Work out the finished part from the listing and answer in its coordinate system (mm). Face numbers are marked on the shaded views. A direction names the side the tool comes from. Coordinates: 2 decimals unless noted, no trailing zeros. Order: outer loops, then holes, each group sorted by start corner. A loop starts at its lowest first (then second) coordinate and runs counter-clockwise, first axis right, second up. Notation, with made-up numbers: (67, 25.25) -> (77, 25.25) arc R15 cw to (77, 37.25) -> close; hole circle Ø4 at (44, 7). An arc over 180 degrees is marked (long way). Answer as CSV lines item,"result". Start each with the question number.
Item 1: Straight lines are drawn through the part: L1, parallel to X at y = 2, z = 28; L2, parallel to Y at x = -7, z = 18.75; L3, parallel to X at y = 5, z = 4. For each, find the intervals that lie inside material, in ascending order.
Item 2: Section A-A (y = 0) is taken. Write down the section's boundary in (x, z).
Item 3: Each of these flat-tipped pins is pushed along its axis until it touches: pin 1 Ø16.5 at (y, z) = (-4, 21) entering from +X; pin 2 Ø1.5 at (y, z) = (-15.5, 19) entering from -X; pin 3 Ø4.5 at (y, z) = (-7, 8.5) entering from -X. Where does it stop, or does it pass through?
Item 4: Section C-C (z = 7.25) is taken. Count the separate pieces of the cut face and the enclosed holes in it, then the cut area to 3 significant figures.
Item 5: Which of the six approach directions +Z, -Z, +X, -X, +Y, -Y give full straight-line access (tool end or side, diameter ignored) to the marked faces 4, 5 and 6?
Item 6: For a pull along X with two mould halves and no side action, classify the marked faces 1, 2 and 3 as pulls with the +X half, pulls with the -X half, needs draft (parallel to the pull), parting line crosses it, or undercut.
Item 7: Section D-D (y = -15) is taken. Write down the section's boundary in (x, z), then the cut area to 3 significant figures.
Item 8: Section B-B (x = -5) is taken. Write down the section's boundary in (y, z), then the cut area to 3 significant figures.
```python
from build123d import *

# Parameters (mm, degrees)
SKETCH_1_W      = 15
SKETCH_1_H      = 25.166666667
EXTRUDE_1_DEPTH = 30
FILLET_1_R      = 5
FILLET_2_R      = 5
FILLET_3_R      = 5


with BuildPart() as part:
    # 草圖1 → 填料-伸長1 (new body)
    with BuildSketch(Plane.XY):
        Polygon((-23.5, 11.416666667), (51.5, 11.416666667), (51.5, 8.416666667), (46.5, 8.416666667), (46.5, -16.75), (51.5, -16.75), (51.5, -19.75), (-23.5, -19.75), (-23.5, -17.25), (-18.5, -17.25), (-18.5, 7.916666667), (-23.5, 7.916666667), align=None)
        with Locations((-6, -4.166666666)):
            Rectangle(SKETCH_1_W, SKETCH_1_H, mode=Mode.SUBTRACT)
        with Locations((14, -4.166666666)):
            Rectangle(SKETCH_1_W, SKETCH_1_H, mode=Mode.SUBTRACT)
        with Locations((34, -4.166666666)):
            Rectangle(SKETCH_1_W, SKETCH_1_H, mode=Mode.SUBTRACT)
    extrude(amount=EXTRUDE_1_DEPTH)

    # 圓角1
    fillet_1_edges = [part.edges().sort_by_distance(p)[0] for p in [
        (-18.5, 7.916666667, 15),
    ]]
    fillet(fillet_1_edges, radius=FILLET_1_R - 0.0001)  # a hair under: the kernel refuses the full size

    # 圓角2
    fillet_2_edges = [part.edges().sort_by_distance(p)[0] for p in [
        (-18.5, -17.25, 15),
    ]]
    fillet(fillet_2_edges, radius=FILLET_2_R - 0.0001)  # a hair under: the kernel refuses the full size

    # 圓角3
    fillet_3_edges = [part.edges().sort_by_distance(p)[0] for p in [
        (46.5, 8.416666667, 15),
        (46.5, -16.75, 15),
        (-13.5, 8.416666667, 15),
        (-13.5, -16.75, 15),
        (1.5, -16.75, 15),
        (1.5, 8.416666667, 15),
        (6.5, 8.416666667, 15),
        (6.5, -16.75, 15),
        (21.5, -16.75, 15),
        (21.5, 8.416666667, 15),
        (26.5, 8.416666667, 15),
        (26.5, -16.75, 15),
        (41.5, -16.75, 15),
        (41.5, 8.416666667, 15),
    ]]
    fillet(fillet_3_edges, radius=FILLET_3_R - 0.0001)  # a hair under: the kernel refuses the full size


solid = part.part
```
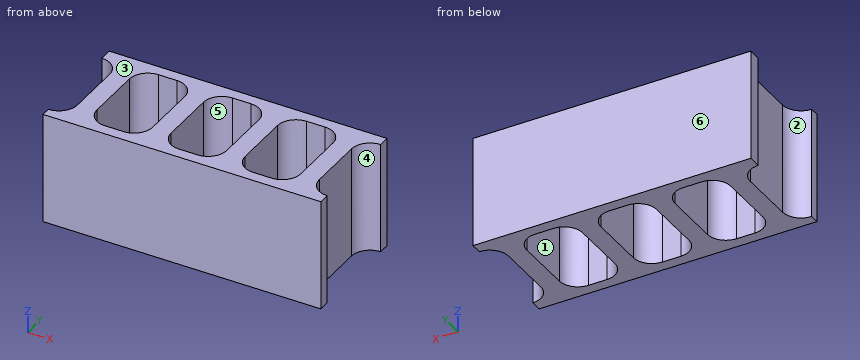
Checked values:
1,L1,"x = -18.5 to -13.5, 1.5 to 6.5, 21.5 to 26.5, 41.5 to 46.5"
1,L2,"y = -19.75 to -16.75, 8.42 to 11.42"
1,L3,"x = -18.95 to -13.24, 1.24 to 6.76, 21.24 to 26.76, 41.24 to 46.76"
2,outline,"(-18.5, 0) -> (-13.5, 0) -> (-13.5, 30) -> (-18.5, 30) -> close; (1.5, 0) -> (6.5, 0) -> (6.5, 30) -> (1.5, 30) -> close; (21.5, 0) -> (26.5, 0) -> (26.5, 30) -> (21.5, 30) -> close; (41.5, 0) -> (46.5, 0) -> (46.5, 30) -> (41.5, 30) -> close"
3,pin 1,"stops at x = 46.57"
3,pin 2,"stops at x = -20.5"
3,pin 3,"stops at x = -18.5"
4,separate pieces,"1"
4,enclosed holes,"3"
4,area,"1,040 mm^2"
5,face 4,"+Z, -Z, +X"
5,face 5,"+Z, -Z"
5,face 6,"+Z, -Z, +X, -X, +Y"
6,face 1,"undercut"
6,face 2,"pulls with the -X half"
6,face 3,"needs draft"
7,outline,"(-19.32, 0) -> (-12.3, 0) -> (-12.3, 30) -> (-19.32, 30) -> close; (0.3, 0) -> (7.7, 0) -> (7.7, 30) -> (0.3, 30) -> close; (20.3, 0) -> (27.7, 0) -> (27.7, 30) -> (20.3, 30) -> close; (40.3, 0) -> (47.7, 0) -> (47.7, 30) -> (40.3, 30) -> close"
7,area,"877 mm^2"
8,outline,"(-19.75, 0) -> (-16.75, 0) -> (-16.75, 30) -> (-19.75, 30) -> close; (8.42, 0) -> (11.42, 0) -> (11.42, 30) -> (8.42, 30) -> close"
8,area,"180 mm^2"
